CAD build for the part. Positions are in the model's coordinates, mm. Give positions to 0.01 mm unless a question says otherwise; leave off trailing zeros. Loops run counter-clockwise (first coordinate to the right, second up) from the corner with the lowest first, then second, coordinate; pieces in that order, holes last.
Item 1: Saw through at A-A on z = 1.55. Give the number of separate pieces and of enclosed holes in the cut face, plus the area to 3 significant figures.
Item 2: Probe probe 1 along X at (y, z) = (24.5, 2.85); probe 2 along X at (y, z) = (26.5, 2.8). List the from-to ranges inside material, lowest first.
Item 3: Saw through at B-B on y = 11.25. Give the cut face in (x, z), plus the area to 3 significant figures.
Item 4: Drop flat-ended pins along their axis: P1, Ø2.5, axis at x = 19.42, y = 21.35, coming from the +Z side; P2, Ø2, axis at y = 26, z = 3, coming from the +X side. Give the stop position or say it passes through.
Solid Edge part; units mm, degrees
sketch "Sketch1" plane through (0, 0, 0) normal (0, 0, 1) x (1, 0, 0)
  line L0 (4.4214, 6.3508) -> (254.4214, 6.3508)
  line L1 (254.4214, 6.3508) -> (254.4214, 36.3508)
  line L2 (254.4214, 36.3508) -> (4.4214, 36.3508)
  line L3 (4.4214, 36.3508) -> (4.4214, 6.3508)
extrude "Protrusion1" add sketch "Sketch1" along normal blind 4
fillet "Redondo_1" radius 15 4 edges at (254.4214, 6.3508, 2) (254.4214, 36.3508, 2) (4.4214, 6.3508, 2) (4.4214, 36.3508, 2)
hole "Furo_8" at (19.4214, 21.3508, 4) direction (0, 0, -1) diameter 3 end up to next
hole "Hole1" at (239.4214, 21.3508, 4) direction (0, 0, -1) diameter 3 end up to next
Results below:
1. separate pieces: 1
1. enclosed holes: 2
1. area: 7,290 mm2
2. probe 1: x = 4.76 to 254.09
2. probe 2: x = 5.33 to 253.51
3. outline: (8.33, 0) - (250.51, 0) - (250.51, 4) - (8.33, 4) - close
3. area: 969 mm2
4. P1: passes through
4. P2: stops at x = 253.97
